Autodesk Inventor part; units mm, degrees
ref_plane "YZ Plane" through (0, 0, 0) normal (1, 0, 0) x (0, 1, 0)
ref_plane "XZ Plane" through (0, 0, 0) normal (0, 1, 0) x (-1, 0, 0)
ref_plane "XY Plane" through (0, 0, 0) normal (0, 0, 1) x (1, 0, 0)
sketch "Szkic7" plane through (0, 0, 0) normal (0, 1, 0) x (-1, 0, 0)
  line L0 (0, -49) -> (0, 49)
  line L1 (35, 0) -> (-35, 0)
  line L2 (15, 25) -> (-15, 25)
  line L3 (-15, 25) -> (-15, -25)
  line L4 (-15, -25) -> (15, -25)
  line L5 (15, -25) -> (15, 25)
  line L6 (15, 25) -> (-15, -25) construction
  line L7 (-15, 25) -> (15, -25) construction
  line L8 (25, 35) -> (-25, 35)
  line L9 (-25, 35) -> (-25, -35)
  line L10 (-25, -35) -> (25, -35)
  line L11 (25, -35) -> (25, 35)
  line L12 (25, 35) -> (-25, -35) construction
  line L13 (-25, 35) -> (25, -35) construction
  line L14 (-15, 25) -> (-15, 35)
  line L15 (-15, -25) -> (-15, -35)
  point P0 (0, 0)
  dimension "d40" = 30
  dimension "d41" = 50
  dimension "d42" = 50
  dimension "d43" = 70
extrude "Wyciągnięcie proste6" add sketch "Szkic7" along normal blind 10 contours L10 L15 L4 L0 | L0 L4 L5 L1 L11 L10 | L10 L9 L1 L3 L15 | L1 L5 L2 L0 L8 L11 | L2 L14 L8 L0 | L1 L9 L8 L14 L3
extrude "Wyciągnięcie proste7" add sketch "Szkic7" along normal blind 50 contours L10 L9 L1 L3 L15 | L1 L9 L8 L14 L3
sketch "Szkic8" plane through (25, 0, 35) normal (1, 0, 0) x (0, 0, -1)
  line L0 (0, 10) -> (70, 10)
  line L1 (70, 10) -> (70, 50)
  line L2 (70, 50) -> (0, 50)
  line L3 (0, 50) -> (0, 10)
  line L4 (35, 50) -> (35, 10)
  circle A0 centre (48, 30) radius 8.1
  line L5 (48, 30) -> (35, 30)
  circle A1 centre (22, 30) radius 8.1
  line L6 (29.65, 46.662236) -> (40.35, 46.662236)
  line L7 (40.35, 46.662236) -> (40.35, 32.662236)
  line L8 (40.35, 32.662236) -> (29.65, 32.662236)
  line L9 (29.65, 32.662236) -> (29.65, 46.662236)
  line L10 (29.65, 46.662236) -> (40.35, 32.662236) construction
  line L11 (40.35, 46.662236) -> (29.65, 32.662236) construction
  circle A2 centre (32.15, 44.162236) radius 1.5
  line L12 (29.65, 44.162236) -> (30.65, 44.162236) construction
  line L13 (32.15, 46.662236) -> (32.15, 45.662236) construction
  line L14 (35, 32.662236) -> (35, 35.202236)
  line L15 (35, 35.202236) -> (40.35, 35.202236)
  line L16 (35, 35.202236) -> (29.65, 35.202236)
  circle A3 centre (32.15, 44.162236) radius 2.5 construction
  line L17 (29.65, 42.71886) -> (32.15, 41.275485)
  line L18 (32.15, 41.275485) -> (34.65, 42.71886)
  line L19 (29.65, 42.71886) -> (29.65, 45.605612)
  line L20 (29.65, 45.605612) -> (32.15, 47.048987)
  line L21 (32.15, 47.048987) -> (34.65, 45.605612)
  line L22 (34.65, 45.605612) -> (34.65, 42.71886)
  line L23 (12, 40.5) -> (58, 40.5)
  line L24 (58, 40.5) -> (58, 19.5)
  line L25 (58, 19.5) -> (12, 19.5)
  line L26 (12, 19.5) -> (12, 40.5)
  line L27 (12, 40.5) -> (58, 19.5) construction
  line L28 (58, 40.5) -> (12, 19.5) construction
  point P0 (35, 39.662236)
  point P1 (9.59459, 19.012494)
  point P2 (9.59459, 19.012494)
  point P3 (12.764463, 33.012494)
  point P4 (11.424717, 33.012494)
  point P5 (9.59459, 29.069118)
  point P6 (32.819873, 46.662236)
  point P7 (31.480127, 46.662236)
  dimension "d62" = 16.2
  dimension "d63" = 13
  dimension "d64" = 10.7
  dimension "d65" = 14
  dimension "d66" = 3
  dimension "d67" = 1
  dimension "d68" = 1
  dimension "d69" = 2.54
  dimension "d70" = 5
  dimension "d71" = 120
  dimension "d72" = 120
  dimension "d73" = 120
  dimension "d74" = 120
  dimension "d75" = 120
  dimension "d76" = 40
  dimension "d77" = 46
  dimension "d78" = 21
extrude "Wyciągnięcie proste8" cut sketch "Szkic8" against normal through all contours A1 | L25 L26 L23 L9 L8 L4 | L4 L5 A0 L7 L23 L24 L25 | L4 L8 A0 L5 | L8 L9 L16 L4 | L4 L15 L7 L8 | A0 | L23 L7 L15 L4 | L4 L16 L9 L23 | L21 L22 L18 L17 L9 L20 L6 | L6 L20 L21 | A2
extrude "Wyciągnięcie proste9" add sketch "Szkic8" against normal blind 7 contours L25 L26 L23 L9 L8 L4 | L4 L5 A0 L7 L23 L24 L25 | L4 L8 A0 L5 | L23 L7 L15 L4 | L4 L16 L9 L23 | L21 L22 L18 L17 L9 L20 L6 | L6 L20 L21
extrude "Wyciągnięcie proste10" cut sketch "Szkic8" against normal blind 3 contours L6 L7 L23 L4 | L4 L23 L9 L17 L18 L22 L21 L6 | L23 L7 L15 L4 | L4 L16 L9 L23 | L21 L22 L18 L17 L9 L20 L6 | L20 L9 L6
extrude "Wyciągnięcie proste11" add sketch "Szkic7" against normal blind 20 contours L10 L15 L4 L0 | L0 L4 L5 L1 L11 L10 | L10 L9 L1 L3 L15 | L1 L5 L2 L0 L8 L11 | L2 L14 L8 L0 | L1 L9 L8 L14 L3
properties part number "uMule-UDaR-sensor"
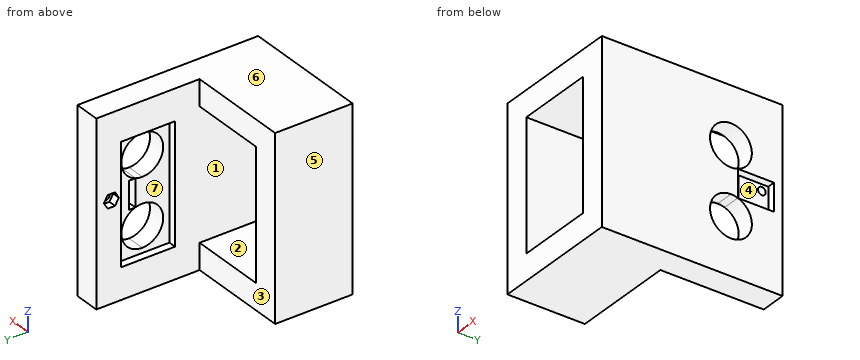
Model file for the job. Use its own axes, mm. Face numbers are marked on the shaded views. A direction names the side the tool comes from. Give positions to 0.01 mm unless a question says otherwise; leave off trailing zeros. Loops run counter-clockwise (first coordinate to the right, second up) from the corner with the lowest first, then second, coordinate; pieces in that order, holes last. Notation, with made-up numbers: (20.5, -27.75) -> (63.5, -27.75) arc R8 cw to (63.5, -19.75) -> close; hole circle Ø9 at (39, 64). An arc over 180 degrees is marked (long way). Use a Markdown table: item, result. Add a question column.
(1) Drop flat-ended pins along their axis: pin 1 Ø6.5 at (y, z) = (28, -8) entering from -X; pin 2 Ø21 at (y, z) = (31.5, 7) entering from -X. Give the stop position or say it passes through.
(2) Slice it at D-D on z = 30.5. List the corners of the cut face in (x, y), and give its area (3 significant figures).
(3) Mould opens along Z. For the marked faces 5, 6 and 7 say: +Z half, -Z half, draft (parallel to the pull), parting line (faces both ways), or undercut.
(4) Slice it at C-C on y = 2.5. List the corners of the cut face in (x, z), and give its area (3 significant figures).
(5) Slice it at A-A on z = 13. List the corners of the cut face in (x, y).
(6) Slice it at B-B on x = -5. List the corners of the cut face in (y, z).
(7) Tool access for the marked faces 1, 2, 3 and 4: list every direction of +Z, -Z, +X, -X, +Y, -Y with a clear straight run to the whole face (end or side of a thin tool).
(8) Wall check: line 1 along Z through (x, y) = (22, 30); line 2 along Y through (x, z) = (19.8, 2.85); line 3 along Z through (x, y) = (5, -7). Give the ranges that are in metal, low to high.
Filled sheet:
| question | item | result |
|---|---|---|
| 1 | pin 1 | x = 18 |
| 1 | pin 2 | x = 15 |
| 2 | outline | (-25, -20) -> (25, -20) -> (25, 50) -> (15, 50) -> (15, 10) -> (-25, 10) -> close |
| 2 | area | 1,900 mm2 |
| 3 | face 5 | draft |
| 3 | face 6 | +Z half |
| 3 | face 7 | undercut |
| 4 | outline | (-25, -35) -> (25, -35) -> (25, 35) -> (-25, 35) -> close; hole (-15, -25) -> (15, -25) -> (15, 25) -> (-15, 25) -> close |
| 4 | area | 2,000 mm2 |
| 5 | outline | (-25, -20) -> (-15, -20) -> (-15, 10) -> (-25, 10) -> close; (15, -20) -> (25, -20) -> (25, 21.9) -> (18, 21.9) -> (18, 19.5) -> (15, 19.5) -> close; (15, 40.5) -> (18, 40.5) -> (18, 38.1) -> (25, 38.1) -> (25, 50) -> (15, 50) -> close |
| 6 | outline | (-20, -35) -> (10, -35) -> (10, -25) -> (-20, -25) -> close; (-20, 25) -> (10, 25) -> (10, 35) -> (-20, 35) -> close |
| 7 | face 1 | +Y |
| 7 | face 2 | +Y, -Y |
| 7 | face 3 | +Z, -Z, -X, +Y |
| 7 | face 4 | +X |
| 8 | line 1 | -35 to -21.1, -4.9 to 4.9, 21.1 to 35 |
| 8 | line 2 | -20 to 32.66, 35.2 to 42.66, 45.66 to 50 |
| 8 | line 3 | -35 to -25, 25 to 35 |
